```python
from build123d import *

# Parameters (mm, degrees)
F0_W     = 10
F0_H     = 91.1132134497
F0_W_2   = 10.2482907567
F0_H_2   = 10
F0_W_3   = 10.1232041232
F0_H_3   = 90.4400162399
F0_W_4   = 146.2950482965
F1_DEPTH = 20
F2_DEPTH = 25
F3_DEPTH = 40


with BuildPart() as f1:
    # F0 (on Top) → F1 (new body)
    with BuildSketch(Plane.XY):
        Polygon((90, 45.8233915269), (100, 45.8233915269), (100, 70), (74.6184438467, 70), (74.6184438467, 60), (90, 60), align=None)
        with Locations((95, 0.2667848021)):
            Rectangle(F0_W, F0_H)
        Polygon((79.7517092433, -60), (90, -60), (90, -45.2898219228), (90, 45.8233915269), (90, 60), (74.6184438467, 60), (-71.6766044497, 60), (-90, 60), (-90, 45.8233915269), (-90, -44.6166247129), (-90, -60), (-79.8767958768, -60), (-79.8767958768, -50), (-80, -50), (-80, 50), (80, 50), (80, -50), (79.7517092433, -50), align=None)
        Polygon((90, -70), (100, -70), (100, -45.2898219228), (90, -45.2898219228), (90, -60), align=None)
        with Locations((84.8758546216, -65)):
            Rectangle(F0_W_2, F0_H_2)
        Polygon((-100, -70), (-90, -70), (-90, -60), (-90, -44.6166247129), (-100, -44.6166247129), align=None)
        with Locations((-84.9383979384, -65)):
            Rectangle(F0_W_3, F0_H_2)
        with Locations((-95, 0.603383407)):
            Rectangle(F0_W, F0_H_3)
        Polygon((-71.6766044497, 60), (-71.6766044497, 70), (-100, 70), (-100, 45.8233915269), (-90, 45.8233915269), (-90, 60), align=None)
        with Locations((1.4709196985, 65)):
            Rectangle(F0_W_4, F0_H_2)
    extrude(amount=F1_DEPTH)

    # F0 (on Top) → F2 (join)
    with BuildSketch(Plane.XY):
        Polygon((-71.6766044497, 60), (-71.6766044497, 70), (-100, 70), (-100, 45.8233915269), (-90, 45.8233915269), (-90, 60), align=None)
        with Locations((-95, 0.603383407)):
            Rectangle(F0_W, F0_H_3)
        Polygon((-100, -70), (-90, -70), (-90, -60), (-90, -44.6166247129), (-100, -44.6166247129), align=None)
        with Locations((1.4709196985, 65)):
            Rectangle(F0_W_4, F0_H_2)
        Polygon((90, 45.8233915269), (100, 45.8233915269), (100, 70), (74.6184438467, 70), (74.6184438467, 60), (90, 60), align=None)
        with Locations((95, 0.2667848021)):
            Rectangle(F0_W, F0_H)
        Polygon((90, -70), (100, -70), (100, -45.2898219228), (90, -45.2898219228), (90, -60), align=None)
    extrude(amount=F2_DEPTH)

    # F0 (on Top) → F3 (join)
    with BuildSketch(Plane.XY):
        Polygon((-71.6766044497, 60), (-71.6766044497, 70), (-100, 70), (-100, 45.8233915269), (-90, 45.8233915269), (-90, 60), align=None)
        Polygon((-100, -70), (-90, -70), (-90, -60), (-90, -44.6166247129), (-100, -44.6166247129), align=None)
        with Locations((-84.9383979384, -65)):
            Rectangle(F0_W_3, F0_H_2)
        with Locations((84.8758546216, -65)):
            Rectangle(F0_W_2, F0_H_2)
        Polygon((90, -70), (100, -70), (100, -45.2898219228), (90, -45.2898219228), (90, -60), align=None)
        Polygon((90, 45.8233915269), (100, 45.8233915269), (100, 70), (74.6184438467, 70), (74.6184438467, 60), (90, 60), align=None)
    extrude(amount=-F3_DEPTH)


solid = f1.part
```
Design review of the part built by this model. Coordinates are the model's own, in mm. A direction names the side the tool comes from. Coordinates: 2 decimals unless noted, no trailing zeros. Write each loop counter-clockwise with the first axis right and the second up, starting at its lowest first coordinate (ties: lowest second). Pieces come first, ordered by that corner, then holes.
1) Mouldability with a two-part tool opening along X and no side actions: class faces 1 (the flat face through (82, 60, -20)), 2 (the flat face through (100, -1, 6)), 3 (the flat face through (1, 70, 7)) as +X half, -X half, draft (parallel to the pull), parting line (faces both ways), or undercut.
2) To check wall thickness, follow L1, parallel to X at y = -30, z = 7; L2, parallel to Y at x = 89, z = -14; L3, parallel to X at y = 56.5, z = -10. State the ranges of each line that lie inside material, in increasing order.
3) Insertion check: pin 1 (5.5 mm diameter, centred on x = -21.5, z = 23.5, fed in from -Y). The pin has a flat end and moves straight along its axis. Give the tip position at first contact, or say it passes through.
4) Add section A-A (z = -13.5). Write out the cut boundary in (x, y), plus the area to 3 significant figures.
5) Add section C-C (x = -55). Write out the cut boundary in (y, z), plus the area to 3 significant figures.
6) Add section D-D (z = 5). Write out the cut boundary in (x, y).
7) Machinability: for faces 4 (the flat face through (-90, -6, 22)), 5 (the flat face through (74.618, 65, -20)), 6 (the flat face through (79.752, -62, -4)), 7 (the flat face through (80, 1, 10)), 8 (the flat face through (-85, -60, -20)), which of the approach directions +Z, -Z, +X, -X, +Y, -Y give a long, thin tool a straight path to every point of the face, cutting with its end or side? Answer none if there is none.
8) Add section B-B (y = -54). Write out the cut boundary in (x, z), plus the area to 3 significant figures.
Check result:
1. face 1: undercut
1. face 2: +X half
1. face 3: draft
2. L1: x = -100 to -80, 80 to 100
2. L2: y = -70 to -60, 60 to 70
2. L3: x = -100 to -90, 90 to 100
3. pin 1: stops at y = 60
4. outline: (-100, -70) - (-79.88, -70) - (-79.88, -60) - (-90, -60) - (-90, -44.62) - (-100, -44.62) - close; (-100, 45.82) - (-90, 45.82) - (-90, 60) - (-71.68, 60) - (-71.68, 70) - (-100, 70) - close; (74.62, 60) - (90, 60) - (90, 45.82) - (100, 45.82) - (100, 70) - (74.62, 70) - close; (79.75, -70) - (100, -70) - (100, -45.29) - (90, -45.29) - (90, -60) - (79.75, -60) - close
4. area: 1,530 mm2
5. outline: (50, 0) - (70, 0) - (70, 25) - (60, 25) - (60, 20) - (50, 20) - close
5. area: 450 mm2
6. outline: (-100, -70) - (-79.88, -70) - (-79.88, -50) - (-80, -50) - (-80, 50) - (80, 50) - (80, -50) - (79.75, -50) - (79.75, -70) - (100, -70) - (100, 70) - (-100, 70) - close
7. face 4: +Z, -Y
7. face 5: -Z, +Y, -Y
7. face 6: +Z, -Z, -Y
7. face 7: +Z, -Z
7. face 8: -Z
8. outline: (-100, -40) - (-90, -40) - (-90, 0) - (-79.88, 0) - (-79.88, 20) - (-90, 20) - (-90, 25) - (-100, 25) - close; (79.75, 0) - (90, 0) - (90, -40) - (100, -40) - (100, 25) - (90, 25) - (90, 20) - (79.75, 20) - close
8. area: 1,710 mm2
